```python
from build123d import *

# Parameters (mm, degrees)
F7_W      = 203.2
F7_H      = 254
F8_DEPTH  = 127
F9_T      = -6.35
F10_DEPTH = 25.4


with BuildPart() as f8:
    # F7 (on offset) → F8 (new body)
    with BuildSketch(Plane.XY.offset(127)):
        Rectangle(F7_W, F7_H)
    extrude(amount=F8_DEPTH)

    # F9
    f9_openings = [f8.faces().sort_by_distance(p)[0] for p in [
        (0, 0, 254),
        (0, 0, 127),
    ]]
    offset(amount=F9_T, openings=f9_openings)

    # F10 (cut): a face of the model
    f10_faces = [f8.faces().sort_by_distance(p)[0] for p in [
        (-95.25, 0, 190.5),
    ]]
    extrude(f10_faces, amount=-F10_DEPTH, mode=Mode.SUBTRACT)


solid = f8.part
```
Input: part model. Units: mm. Frame: model coordinates. A direction names the side the tool comes from. Coordinates: 2 decimals unless noted, no trailing zeros. Loops run counter-clockwise (first coordinate to the right, second up) from the corner with the lowest first, then second, coordinate; pieces in that order, holes last. Notation, with made-up numbers: M 7.5,3 L 31.5,3 A21 ccw 31.5,14 Z; hole C 24.25,26.5 d8. An arc over 180 degrees is marked long. One line per item, written item: value.
(1) Reachability of faces 1 (the flat face through (-5, 120.65, 190)), 2 (the flat face through (-1, 127, 190)) from +Z, -Z, +X, -X, +Y, -Y: full face, straight path, thin tool, end or side. Return the list, or none.
Filled in:
face 1: +Z, -Z, -X
face 2: +Z, -Z, +X, -X, +Y
(2) Pin query (flat end, axial travel): pin 1 (1 mm diameter, centred on y = 24, z = 182.5, fed in from -X). Return the tip coordinate at first contact, or that it passes through.
Filled in:
pin 1: x = 95.25
(3) Pull-direction query (Y, two-part tool) for faces 3 (the flat face through (97, 1, 127)), 4 (the flat face through (-1, -127, 190)), 5 (the flat face through (-2, -120.65, 191)); classes: +Y half, -Y half, draft (parallel to the pull), parting line (faces both ways), or undercut.
Filled in:
face 3: draft
face 4: -Y half
face 5: undercut
(4) Section C-C (y = 66). Output: boundary loops of the cut face in (x, z).
Filled in:
outline: M 95.25,127 L 101.6,127 L 101.6,254 L 95.25,254 Z
(5) Line query: line 1 along Y through (x, z) = (-25, 219); line 2 along X through (y, z) = (-88.5, 204). Output: solid intervals per line, ascending. Write a range as from..to.
Filled in:
line 1: -127..-120.65, 120.65..127
line 2: 95.25..101.6
(6) Section A-A (x = 52.5). Output: boundary loops of the cut face in (y, z).
Filled in:
outline: M -127,127 L -120.65,127 L -120.65,254 L -127,254 Z; M 120.65,127 L 127,127 L 127,254 L 120.65,254 Z
(7) Section B-B (z = 232). Output: boundary loops of the cut face in (x, y).
Filled in:
outline: M -101.6,-127 L 101.6,-127 L 101.6,127 L -101.6,127 L -101.6,120.65 L 95.25,120.65 L 95.25,-120.65 L -101.6,-120.65 Z
